from build123d import *

# Parameters (mm, degrees)
BOSS_EXTRUDE2_DEPTH   = 6
SKETCH3_W             = 2.51964915
SKETCH3_H             = 4
BOSS_EXTRUDE2_2_DEPTH = 6
LPATTERN1_COUNT       = 5
LPATTERN1_PITCH       = 2
SKETCH4_W             = 10.51964915
SKETCH4_H             = 8.85
BOSS_EXTRUDE3_DEPTH   = 3
BOSS_EXTRUDE7_DEPTH   = 3
BOSS_EXTRUDE8_START   = -3
BOSS_EXTRUDE8_DEPTH   = 2
BOSS_EXTRUDE9_START   = -5
BOSS_EXTRUDE9_DEPTH   = 4
FILLET1_R             = 1


with BuildPart() as part:
    # Sketch3 → Boss-Extrude2 (new body)
    with BuildSketch(Plane(origin=(0, 0, 0), x_dir=(-1, 0, 0), z_dir=(0, 1, 0))):
        with BuildLine():
            Line((0, 0.425), (0.51964915, 0.425))
            ThreePointArc((0.51964915, 0.425), (0.618556221, 0.462228588), (0.668367684, 0.555434783))
            ThreePointArc((0.668367684, 0.555434783), (0.702212861, 0.713062154), (0.76094817, 0.863202247))
            ThreePointArc((0.76094817, 0.863202247), (1.259824575, 1.175), (1.758700979, 0.863202247))
            ThreePointArc((1.758700979, 0.863202247), (1.817436289, 0.713062154), (1.851281466, 0.555434783))
            ThreePointArc((1.851281466, 0.555434783), (1.901092929, 0.462228588), (2, 0.425))
            Line((2, 0.425), (2.51964915, 0.425))
            Line((2.51964915, 0.425), (2.51964915, 4.425))
            Line((2.51964915, 4.425), (0, 4.425))
            Line((0, 4.425), (0, 0.425))
        make_face()
    boss_extrude2 = extrude(amount=BOSS_EXTRUDE2_DEPTH)


with BuildPart() as body_2:
    # Sketch3 → Boss-Extrude2 2 (new body)
    with BuildSketch(Plane(origin=(0, 0, 0), x_dir=(-1, 0, 0), z_dir=(0, 1, 0))):
        with Locations((1.259824575, -2.425)):
            Rectangle(SKETCH3_W, SKETCH3_H)
    boss_extrude2_2 = extrude(amount=BOSS_EXTRUDE2_2_DEPTH)


with BuildPart() as part_1:
    add(part.part)

    add(body_2.part)  # LPattern1 merges body 2
    # LPattern1: Boss-Extrude2, Boss-Extrude2 2 ×5
    with Locations(*[(i * LPATTERN1_PITCH, 0, 0) for i in range(1, LPATTERN1_COUNT)]):
        add(boss_extrude2)
        add(boss_extrude2_2)

    # Sketch4 → Boss-Extrude3 (add)
    with BuildSketch(Plane(origin=(0, 6, 0), x_dir=(1, 0, 0), z_dir=(0, 1, 0))):
        with Locations((2.740175425, 0)):
            Rectangle(SKETCH4_W, SKETCH4_H)
    extrude(amount=BOSS_EXTRUDE3_DEPTH)

    # Sketch8 → Boss-Extrude7 (add)
    with BuildSketch(Plane(origin=(0, 9, 0), x_dir=(1, 0, 0), z_dir=(0, 1, 0))):
        with BuildLine():
            Line((-2.51964915, 4.425), (-9.714377865, 4.425))
            ThreePointArc((-9.714377865, 4.425), (-9.31964915, 0), (-9.714377865, -4.425))
            Line((-9.714377865, -4.425), (-2.51964915, -4.425))
            Line((-2.51964915, -4.425), (-2.51964915, 4.425))
        make_face()
    extrude(amount=-BOSS_EXTRUDE7_DEPTH)

    # Sketch8<3> → Boss-Extrude8 (add)
    with BuildSketch(Plane(origin=(0, 9, 0), x_dir=(1, 0, 0), z_dir=(0, 1, 0)).offset(BOSS_EXTRUDE8_START)):
        with BuildLine():
            ThreePointArc((-7.279320472, -4.425), (-6.91964915, 0), (-7.279320472, 4.425))
            Line((-7.279320472, 4.425), (-9.714377865, 4.425))
            ThreePointArc((-9.714377865, 4.425), (-9.31964915, 0), (-9.714377865, -4.425))
            Line((-9.714377865, -4.425), (-7.279320472, -4.425))
        make_face()
        with BuildLine():
            Line((-2.51964915, -4.425), (-2.51964915, 4.425))
            Line((-2.51964915, 4.425), (-5.254560555, 4.425))
            ThreePointArc((-5.254560555, 4.425), (-4.91964915, 0), (-5.254560555, -4.425))
            Line((-5.254560555, -4.425), (-2.51964915, -4.425))
        make_face()
    extrude(amount=-BOSS_EXTRUDE8_DEPTH)

    # Sketch8<4> → Boss-Extrude9 (add)
    with BuildSketch(Plane(origin=(0, 9, 0), x_dir=(1, 0, 0), z_dir=(0, 1, 0)).offset(BOSS_EXTRUDE9_START)):
        with BuildLine():
            Line((-2.51964915, 4.425), (-9.714377865, 4.425))
            ThreePointArc((-9.714377865, 4.425), (-9.31964915, 0), (-9.714377865, -4.425))
            Line((-9.714377865, -4.425), (-2.51964915, -4.425))
            Line((-2.51964915, -4.425), (-2.51964915, 4.425))
        make_face()
    extrude(amount=-BOSS_EXTRUDE9_DEPTH)

    # Fillet1
    fillet1_edges = [part_1.edges().sort_by_distance(p)[0] for p in [
        (8, 4.5, 4.425),
        (8, 4.5, -4.425),
        (-9.714377865, 4.5, 4.425),
        (-9.714377865, 4.5, -4.425),
        (-7.279320472, 5, -4.425),
        (-7.279320472, 5, 4.425),
        (-5.254560555, 5, 4.425),
        (-5.254560555, 5, -4.425),
    ]]
    fillet(fillet1_edges, radius=FILLET1_R)


solid = part_1.part
Here's how the part is built. I have some questions about the finished solid (model axes, mm). A direction names the side the tool comes from. Give positions to 0.01 mm unless a question says otherwise; leave off trailing zeros. Order: outer loops, then holes, each group sorted by start corner. A loop starts at its lowest first (then second) coordinate and runs counter-clockwise, first axis right, second up. Notation, with made-up numbers: M 20,5.5 L 54,5.5 A11 ccw 54,21.5 Z; hole C 8.5,-12 d7. An arc over 180 degrees is marked long. Answer as a JSON object with one key per item and string values. Group by question number.
1) We'd pull the mould along Y, two halves only. Please class faces 1 (the flat face through (-6, 6, 0)), 2 (the cylindrical face through (-9.291, 4.563, 4.093)), 3 (the flat face through (-1, 0, -1)): pulls with the +Y half, pulls with the -Y half, needs draft (parallel to the pull), parting line crosses it, or undercut.
2) Suppose I cut it at C-C, the plane x = 3.75. Write out the boundary of the cut face in (y, z) (3 decimals).
3) I'm going to push a flat-ended pin straight in: pin 1 Ø1 at (y, z) = (5, 1) entering from -X. Where does the tip first touch, or does it pass through?
4) Suppose I cut it at B-B, the plane z = 2. Write out the boundary of the cut face in (x, y).
5) Please list where these lines run through material, in increasing order: L1, parallel to Z at x = 3.5, y = 2.25 (3 decimals); L2, parallel to Y at x = 0.25, z = 0.75; L3, parallel to X at y = 7.5, z = 3.25. Write a range as [from, to].
6) Suppose I cut it at A-A, the plane x = -6. Write out the boundary of the cut face in (y, z) (3 decimals).
7) Suppose I cut it at D-D, the plane x = -1. Write out the boundary of the cut face in (y, z) (3 decimals).
8) On a 3-axis mill with a long thin cutter (end or side, diameter ignored), from which of +Z, -Z, +X, -X, +Y, -Y can I reach the whole of each face in a straight line? I mean faces 4 (the cylindrical face through (7.7, 4.56, 4.14)), 5 (the cylindrical face through (-7.49, 4.99, -4.18)), 6 (the flat face through (-2.52, 3, 0)), 7 (the cylindrical face through (-6.92, 5.01, 0.05)), 8 (the cylindrical face through (0.749, 2.958, 1.175)). Say none if no direction works.
Results found:
{
 "1": {"face 1": "undercut", "face 2": "needs draft", "face 3": "pulls with the -Y half"},
 "2": {"outline": "M 0,-4.425 L 9,-4.425 L 9,4.425 L 0,4.425 L 0,0.425 L 6,0.425 L 6,-0.425 L 0,-0.425 Z"},
 "3": {"pin 1": "x = -9.36"},
 "4": {"outline": "M -9.4,0 L 8,0 L 8,9 L -9.4,9 Z; hole M -6.99,4 L -4.99,4 L -4.99,6 L -6.99,6 Z"},
 "5": {"L1": "[-4.425, -0.425], [0.425, 4.425]", "L2": "[6, 9]", "L3": "[-9.53, 8]"},
 "6": {"outline": "M 0,-4.425 L 4,-4.425 L 4,4.425 L 0,4.425 Z; M 6,-4.425 L 9,-4.425 L 9,4.425 L 6,4.425 Z"},
 "7": {"outline": "M 0,-4.425 L 9,-4.425 L 9,4.425 L 0,4.425 L 0,1.11 L 6,1.11 L 6,-0.425 L 0,-0.425 Z"},
 "8": {"face 4": "+Z, +X, +Y, -Y", "face 5": "-Z", "face 6": "+X, -Y", "face 7": "none", "face 8": "-Y"}
}
